For this review, take the finished solid that the model builds, in its own axes (mm). A direction names the side the tool comes from. Give positions to 0.01 mm unless a question says otherwise; leave off trailing zeros. Order: outer loops, then holes, each group sorted by start corner. A loop starts at its lowest first (then second) coordinate and runs counter-clockwise, first axis right, second up. Notation, with made-up numbers: M 88,-26.5 L 119,-26.5 A23 cw 119,-7.5 Z; hole C 76,-18.75 d6. An arc over 180 degrees is marked long. Answer as CSV lines item,"result". Start each with the question number.
1. Machinability: for faces 1 (the flat face through (400, -347, 493)), 2 (the flat face through (197, 150, 493)), 3 (the flat face through (-101, 350, 493)), 4 (the flat face through (344, 8, 0)), 5 (the flat face through (-101, -350, 493)), which of the approach directions +Z, -Z, +X, -X, +Y, -Y give a long, thin tool a straight path to every point of the face, cutting with its end or side? Answer none if there is none.
2. We need section B-B, the plane z = 108.5. Give the boundary of the cut face in (x, y).
3. We need section A-A, the plane y = -240.5. Give the boundary of the cut face in (x, z), and give its area (3 significant figures).
4. We need section D-D, the plane y = 419.5. Give the boundary of the cut face in (x, z).
5. For line 1 along X through (y, z) = (-275, 846.5); line 2 along Y through (x, z) = (229, 564.5); line 3 along Y through (x, z) = (-138, 152), list the stretches that pass through material, from the lowest coordinate up.
6. Mouldability with a two-part tool opening along X and no side actions: class faces 6 (the flat face through (548, -550, 493)), 7 (the flat face through (197, -150, 493)), 8 (the flat face through (-200, -5, 493)) as pulls with the +X half, pulls with the -X half, needs draft (parallel to the pull), parting line crosses it, or undercut.
7. We need section C-C, the plane x = 171.5. Give the boundary of the cut face in (y, z).
Solid Edge part; units mm, degrees
sketch "Sketch1" plane through (0, 0, 0) normal (0, 0, 1) x (1, 0, 0)
  line L0 (400, -150) -> (400, -550)
  line L1 (400, -550) -> (700, -550)
  line L2 (700, -550) -> (700, 0)
  line L3 (700, 550) -> (700, 0)
  line L4 (400, 550) -> (700, 550)
  line L5 (400, 150) -> (400, 550)
  line L6 (0, 150) -> (400, 150)
  line L7 (0, 350) -> (0, 150)
  line L8 (-200, 350) -> (0, 350)
  line L9 (-200, 0) -> (-200, 350)
  line L10 (-200, 0) -> (-200, -350)
  line L11 (-200, -350) -> (0, -350)
  line L12 (0, -350) -> (0, -150)
  line L13 (0, -150) -> (400, -150)
extrude "Protrusion1" add sketch "Sketch1" along normal blind 1000
Result set:
1,face 1,"+Z, -Z, -Y"
1,face 2,"+Z, -Z, +Y"
1,face 3,"+Z, -Z, -X, +Y"
1,face 4,"-Z, +X, -X, +Y, -Y"
1,face 5,"+Z, -Z, -X, -Y"
2,outline,"M -200,-350 L 0,-350 L 0,-150 L 400,-150 L 400,-550 L 700,-550 L 700,550 L 400,550 L 400,150 L 0,150 L 0,350 L -200,350 Z"
3,outline,"M -200,0 L 0,0 L 0,1000 L -200,1000 Z; M 400,0 L 700,0 L 700,1000 L 400,1000 Z"
3,area,"500,000 mm2"
4,outline,"M 400,0 L 700,0 L 700,1000 L 400,1000 Z"
5,line 1,"-200 to 0, 400 to 700"
5,line 2,"-150 to 150"
5,line 3,"-350 to 350"
6,face 6,"needs draft"
6,face 7,"undercut"
6,face 8,"pulls with the -X half"
7,outline,"M -150,0 L 150,0 L 150,1000 L -150,1000 Z"
